from build123d import *

# Parameters (mm, degrees)
BASE_FLANGE1_DEPTH = 12.319
FILLET1_RADIUS     = 12.319
FILLET1_LENGTH     = 2.2352
FILLET2_RADIUS     = 12.319
FILLET2_LENGTH     = 2.2352
SKETCH3_R          = 4.0005
SKETCH3_R_2        = 1.143
EXTRUDE1_DEPTH     = 2.2352
SKETCH5_R          = 4.0005
SKETCH5_R_2        = 1.143
EXTRUDE2_DEPTH     = 2.2352


# Sheet-metal steps are written as plain solids
with BuildPart() as part:
    # Sketch1 → Base-Flange1 (new, symmetric)
    with BuildSketch(Plane(origin=(0, 0, 0), x_dir=(0, 0, -1), z_dir=(1, 0, 0))):
        with BuildLine():
            Line((-28.6258, 0), (-3.048, 0))
            ThreePointArc((-3.048, 0), (-0.892738531, 0.892738531), (0, 3.048))
            Line((0, 3.048), (0, 36.068))
            Line((0, 36.068), (-2.2352, 36.068))
            Line((-2.2352, 36.068), (-2.2352, 3.048))
            ThreePointArc((-2.2352, 3.048), (-2.473263608, 2.473263608), (-3.048, 2.2352))
            Line((-3.048, 2.2352), (-28.6258, 2.2352))
            Line((-28.6258, 2.2352), (-28.6258, 0))
        make_face()
    extrude(amount=BASE_FLANGE1_DEPTH, both=True)

    # Fillet1: full round fillet: the end face becomes a half cylinder, R = half its width
    fillet1_face = Plane((0, 36.068, 1.1176), x_dir=(0, 0, -1), z_dir=(0, 1, 0))  # on the end face: x along it, z out of the body
    fillet1_slab = fillet1_face.offset(-FILLET1_RADIUS / 2) * Box(FILLET1_LENGTH, 2 * FILLET1_RADIUS, FILLET1_RADIUS, mode=Mode.PRIVATE)  # the body's end, R deep
    fillet1_round = Plane((0, 23.749, 1.1176), x_dir=(0, 1, 0), z_dir=(0, 0, -1)) * Cylinder(FILLET1_RADIUS, FILLET1_LENGTH, mode=Mode.PRIVATE)  # its axis R under the face
    add(fillet1_slab - fillet1_round, mode=Mode.SUBTRACT)

    # Fillet2: full round fillet: the end face becomes a half cylinder, R = half its width
    fillet2_face = Plane((0, 1.1176, 28.6258), x_dir=(0, 1, 0), z_dir=(0, 0, 1))  # on the end face: x along it, z out of the body
    fillet2_slab = fillet2_face.offset(-FILLET2_RADIUS / 2) * Box(FILLET2_LENGTH, 2 * FILLET2_RADIUS, FILLET2_RADIUS, mode=Mode.PRIVATE)  # the body's end, R deep
    fillet2_round = Plane((0, 1.1176, 16.3068), x_dir=(0, 0, 1), z_dir=(0, 1, 0)) * Cylinder(FILLET2_RADIUS, FILLET2_LENGTH, mode=Mode.PRIVATE)  # its axis R under the face
    add(fillet2_slab - fillet2_round, mode=Mode.SUBTRACT)

    # Sketch3 → Extrude1 (cut)
    with BuildSketch(Plane.XY.offset(2.2352)):
        with Locations((0, 23.749)):
            Circle(SKETCH3_R)
        with Locations((0, 32.0802)):
            Circle(SKETCH3_R_2)
        with Locations((8.3312, 23.749)):
            Circle(SKETCH3_R_2)
        with Locations((0, 15.4178)):
            Circle(SKETCH3_R_2)
        with Locations((-8.3312, 23.749)):
            Circle(SKETCH3_R_2)
    extrude(amount=-EXTRUDE1_DEPTH, mode=Mode.SUBTRACT)

    # Sketch5 → Extrude2 (cut)
    with BuildSketch(Plane(origin=(0, 2.2352, 0), x_dir=(1, 0, 0), z_dir=(0, 1, 0))):
        with Locations(Location((0, -16.3068, 0), (0, 0, 270))):
            Circle(SKETCH5_R)
        with Locations(Location((0, -7.9756, 0), (0, 0, 270))):
            Circle(SKETCH5_R_2)
        with Locations(Location((8.3312, -16.3068, 0), (0, 0, 270))):
            Circle(SKETCH5_R_2)
        with Locations(Location((0, -24.638, 0), (0, 0, 270))):
            Circle(SKETCH5_R_2)
        with Locations(Location((-8.3312, -16.3068, 0), (0, 0, 270))):
            Circle(SKETCH5_R_2)
    extrude(amount=-EXTRUDE2_DEPTH, mode=Mode.SUBTRACT)


solid = part.part
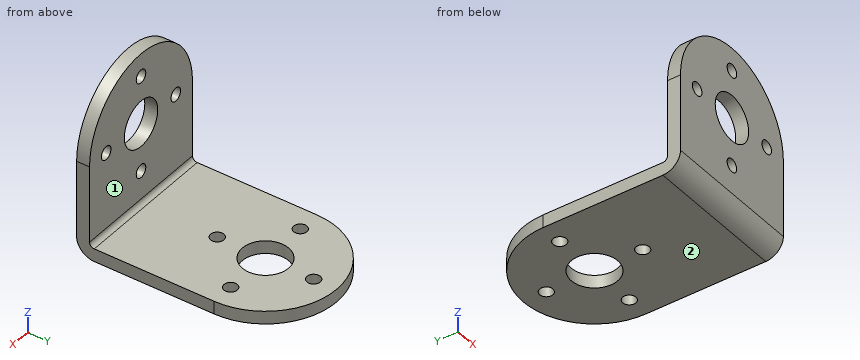
CAD build for the part. Positions are in the model's coordinates, mm. Face numbers are marked on the shaded views. A direction names the side the tool comes from. Give positions to 0.01 mm unless a question says otherwise; leave off trailing zeros. Order: outer loops, then holes, each group sorted by start corner. A loop starts at its lowest first (then second) coordinate and runs counter-clockwise, first axis right, second up. Notation, with made-up numbers: (-2.75, 45) - (8.25, 45) arc R23 cw to (8.25, 74) - close; hole circle Ø1 at (48, 46). An arc over 180 degrees is marked (long way). Write each question's results on one line, items separated by ' | '.
1. Saw through at C-C on x = -2.75. List the corners of the cut face in (y, z), and give its area (3 significant figures).
Calculated:
outline: (0, 3.05) arc R3.05 ccw to (3.05, 0) - (20.84, 0) - (20.84, 2.24) - (3.05, 2.24) arc R0.81 cw to (2.24, 3.05) - (2.24, 13.4) - (0, 13.4) - close; (0, 19.21) - (2.24, 19.21) - (2.24, 28.31) - (0, 28.31) - close; (26.65, 0) - (35.76, 0) - (35.76, 2.24) - (26.65, 2.24) - close | area: 110 mm2
2. Saw through at D-D on z = 25.25. List the corners of the cut face in (x, y), and give its area (3 significant figures).
Calculated:
outline: (-8.47, 0) - (-0.97, 0) - (-0.97, 2.24) - (-8.47, 2.24) - close; (0.97, 0) - (8.47, 0) - (8.47, 2.24) - (0.97, 2.24) - close | area: 33.6 mm2
3. Probe L1, parallel to Z at x = -4, y = 10; L2, parallel to X at y = 22, z = 1.5. List the from-to ranges inside material, lowest first. Write a range as from..to.
Calculated:
L1: z = 0..2.24 | L2: x = -12.32..-3.6, 3.6..12.32
4. Saw through at B-B on y = 26.5. List the corners of the cut face in (x, z), and give its area (3 significant figures).
Calculated:
outline: (-12.01, 0) - (-2.9, 0) - (-2.9, 2.24) - (-12.01, 2.24) - close; (2.9, 0) - (12.01, 0) - (12.01, 2.24) - (2.9, 2.24) - close | area: 40.7 mm2
5. Pin check, flat tips, straight feed: pin 1 (1 mm diameter, centred on x = -5, y = 15, fed in from +Z); pin 2 (3 mm diameter, centred on x = -2, z = 14.5, fed in from +Y). Stop position of each tip, or through.
Calculated:
pin 1: stops at z = 2.24 | pin 2: stops at y = 2.24
6. Saw through at A-A on x = 0. Count the separate pieces of the cut face and the enclosed holes in it, and give its area (3 significant figures).
Calculated:
separate pieces: 7 | enclosed holes: 0 | area: 81.5 mm2
7. 3-axis set-ups, long thin cutter, end or side, ignore diameter. For the marked faces 1 and 2: which of +Z, -Z, +X, -X, +Y, -Y reach the whole face in a straight line?
Calculated:
face 1: +Z, +X, -X, +Y | face 2: -Z, +X, -X, +Y, -Y
